For this review, take the finished solid that the model builds, in its own axes (mm). Face numbers are marked on the shaded views. A direction names the side the tool comes from. Coordinates: 2 decimals unless noted, no trailing zeros. Order: outer loops, then holes, each group sorted by start corner. A loop starts at its lowest first (then second) coordinate and runs counter-clockwise, first axis right, second up.
from build123d import *

# Parameters (mm, degrees)
SKETCH1_W                       = 100
SKETCH1_H                       = 100
BOSS_EXTRUDE1_DEPTH             = 95
SKETCH2_W                       = 10
SKETCH2_H                       = 10
BOSS_EXTRUDE2_DEPTH             = 105
SKETCH3_R                       = 1.4
CUT_EXTRUDE1_DEPTH              = 10
SKETCH4_W                       = 11
SKETCH4_H                       = 11
BOSS_EXTRUDE3_DEPTH             = 105
SKETCH5_R                       = 1.4
CUT_EXTRUDE2_DEPTH              = 10
SKETCH6_R                       = 1.4
CUT_EXTRUDE3_DEPTH              = 10
CHAMFER1_SIZE                   = 1
SKETCH7_W                       = 19
SKETCH7_H                       = 43
SKETCH7_W_2                     = 16
SKETCH7_H_2                     = 40
BOSS_EXTRUDE4_DEPTH             = 3
SKETCH8_W                       = 16
SKETCH8_H                       = 40
CUT_EXTRUDE4_DEPTH              = 10
CHAMFER2_SIZE                   = 13
SKETCH9_W                       = 16
SKETCH9_H                       = 3.1
CUT_EXTRUDE5_DEPTH              = 10
FILLET1_R                       = 1
SKETCH10_R                      = 1.4
CUT_EXTRUDE6_DEPTH              = 10
SKETCH12_W                      = 30.5
SKETCH12_H                      = 2.2
CUT_EXTRUDE7_DEPTH              = 3
SKETCH13_W                      = 30.5
SKETCH13_H                      = 2.2
CUT_EXTRUDE8_DEPTH              = 3
SKETCH14_W                      = 2.2
SKETCH14_H                      = 30.5
CUT_EXTRUDE9_DEPTH              = 3
CUT_EXTRUDE10_DEPTH             = 45
CUT_EXTRUDE10_DEPTH_BACK        = 45
SKETCH15_W                      = 90
SKETCH15_H                      = 58
CUT_EXTRUDE11_REACH             = 125.296
CUT_EXTRUDE11_DIRECTION_2_REACH = 125.296
CHAMFER3_SIZE                   = 4
CUT_EXTRUDE12_DEPTH             = 152.673992497
BOSS_EXTRUDE7_DEPTH             = 10
BOSS_EXTRUDE7_DEPTH_BACK        = 30.5
SKETCH19_W                      = 94
SKETCH19_H                      = 94
SKETCH19_W_2                    = 85
SKETCH19_H_2                    = 85
SKETCH20_R                      = 1.4
CUT_EXTRUDE13_DEPTH             = 123.316188626
SKETCH21_R                      = 1.4
CUT_EXTRUDE14_DEPTH             = 123.316188626
SKETCH22_W                      = 2.2
SKETCH22_H                      = 30.5
BOSS_EXTRUDE8_DEPTH             = 3
SKETCH23_R                      = 1.4
CUT_EXTRUDE15_DEPTH             = 20


with BuildPart() as part:
    # Sketch1 → Boss-Extrude1 (new body)
    with BuildSketch(Plane(origin=(0, 0, 0), x_dir=(1, 0, 0), z_dir=(0, 1, 0))):
        Rectangle(SKETCH1_W, SKETCH1_H)
    extrude(amount=BOSS_EXTRUDE1_DEPTH)

    # Sketch2 → Boss-Extrude2 (add)
    with BuildSketch(Plane(origin=(0, 100, 0), x_dir=(1, 0, 0), z_dir=(0, 1, 0))):
        with Locations((-45, 45)):
            Rectangle(SKETCH2_W, SKETCH2_H)
        with Locations((45, 45)):
            Rectangle(SKETCH2_W, SKETCH2_H)
        with Locations((45, -45)):
            Rectangle(SKETCH2_W, SKETCH2_H)
        with Locations((-45, -45)):
            Rectangle(SKETCH2_W, SKETCH2_H)
    extrude(amount=-BOSS_EXTRUDE2_DEPTH)

    # Sketch3 → Cut-Extrude1 (cut)
    with BuildSketch(Plane(origin=(0, 95, 0), x_dir=(1, 0, 0), z_dir=(0, 1, 0))):
        with Locations(Location((-28, -45, 0), (0, 0, 270))):
            Circle(SKETCH3_R)
        with Locations(Location((28, -45, 0), (0, 0, 90))):
            Circle(SKETCH3_R)
        with Locations(Location((28, 45, 0), (0, 0, 270))):
            Circle(SKETCH3_R)
        with Locations(Location((-28, 45, 0), (0, 0, 90))):
            Circle(SKETCH3_R)
    cut_extrude1 = extrude(amount=-CUT_EXTRUDE1_DEPTH, mode=Mode.SUBTRACT)

    # Sketch4 → Boss-Extrude3 (add)
    with BuildSketch(Plane(origin=(0, 100, 0), x_dir=(1, 0, 0), z_dir=(0, 1, 0))):
        with Locations((-45.5, 45.5)):
            Rectangle(SKETCH4_W, SKETCH4_H)
        with Locations((45.5, 45.5)):
            Rectangle(SKETCH4_W, SKETCH4_H)
        with Locations((45.5, -45.5)):
            Rectangle(SKETCH4_W, SKETCH4_H)
        with Locations((-45.5, -45.5)):
            Rectangle(SKETCH4_W, SKETCH4_H)
    extrude(amount=-BOSS_EXTRUDE3_DEPTH)

    # Sketch5 → Cut-Extrude2 (cut)
    with BuildSketch(Plane.XY.offset(50)):
        with Locations((-36, 91)):
            Circle(SKETCH5_R)
        with Locations(Location((36, 91, 0), (0, 0, 180))):
            Circle(SKETCH5_R)
        with Locations((36, 4)):
            Circle(SKETCH5_R)
        with Locations(Location((-36, 4, 0), (0, 0, 180))):
            Circle(SKETCH5_R)
    cut_extrude2 = extrude(amount=-CUT_EXTRUDE2_DEPTH, mode=Mode.SUBTRACT)

    # Mirror1: Cut-Extrude2 across plane
    add(cut_extrude2.mirror(Plane.XY), mode=Mode.SUBTRACT)

    # Sketch6 → Cut-Extrude3 (cut)
    with BuildSketch(Plane.ZY.offset(50)):
        with Locations((-36, 91)):
            Circle(SKETCH6_R)
        with Locations(Location((36, 91, 0), (0, 0, 180))):
            Circle(SKETCH6_R)
        with Locations((36, 4)):
            Circle(SKETCH6_R)
        with Locations(Location((-36, 4, 0), (0, 0, 180))):
            Circle(SKETCH6_R)
    cut_extrude3 = extrude(amount=-CUT_EXTRUDE3_DEPTH, mode=Mode.SUBTRACT)

    # Mirror2: Cut-Extrude3 across plane
    add(cut_extrude3.mirror(Plane(origin=(0, 0, 0), x_dir=(0, 0, 1), z_dir=(1, 0, 0))), mode=Mode.SUBTRACT)

    # Mirror3: Cut-Extrude1 across plane
    add(cut_extrude1.mirror(Plane.ZX.offset(47.5)), mode=Mode.SUBTRACT)

    # Chamfer1
    chamfer1_edges = [part.edges().sort_by_distance(p)[0] for p in [
        (-45.5, -5, 51),
        (-51, -5, 45.5),
        (-51, 100, 45.5),
        (-45.5, 100, 51),
        (51, -5, 45.5),
        (45.5, -5, 51),
        (45.5, 100, 51),
        (51, 100, 45.5),
        (45.5, -5, -51),
        (51, -5, -45.5),
        (51, 100, -45.5),
        (45.5, 100, -51),
        (-51, -5, -45.5),
        (-45.5, -5, -51),
        (-45.5, 100, -51),
        (-51, 100, -45.5),
        (-45.5, -5, 40),
        (-40, -5, 45.5),
        (-40, 100, 45.5),
        (-45.5, 100, 40),
        (40, -5, 45.5),
        (45.5, -5, 40),
        (45.5, 100, 40),
        (40, 100, 45.5),
        (45.5, -5, -40),
        (40, -5, -45.5),
        (45, 95, -40),
        (40, 100, -45.5),
        (45.5, 100, -40),
        (-40, -5, -45.5),
        (-45.5, -5, -40),
        (-45.5, 100, -40),
        (-40, 100, -45.5),
    ]]
    chamfer(chamfer1_edges, length=CHAMFER1_SIZE)

    # Sketch7 → Boss-Extrude4 (add)
    with BuildSketch(Plane(origin=(0, 95, 0), x_dir=(1, 0, 0), z_dir=(0, 1, 0))):
        with Locations((0, -17)):
            Rectangle(SKETCH7_W, SKETCH7_H)
        with Locations((0, -17)):
            Rectangle(SKETCH7_W_2, SKETCH7_H_2, mode=Mode.SUBTRACT)
    extrude(amount=BOSS_EXTRUDE4_DEPTH)

    # Sketch8 → Cut-Extrude4 (cut)
    with BuildSketch(Plane(origin=(0, 95, 0), x_dir=(1, 0, 0), z_dir=(0, 1, 0))):
        with Locations((0, -17)):
            Rectangle(SKETCH8_W, SKETCH8_H)
    extrude(amount=-CUT_EXTRUDE4_DEPTH, mode=Mode.SUBTRACT)

    # Chamfer2
    chamfer2_edges = [part.edges().sort_by_distance(p)[0] for p in [
        (0, 85, 37),
    ]]
    chamfer(chamfer2_edges, length=CHAMFER2_SIZE - 0.0001)  # a hair under: the kernel refuses the full size

    # Sketch9 → Cut-Extrude5 (cut)
    with BuildSketch(Plane(origin=(0, 85, 0), x_dir=(1, 0, 0), z_dir=(0, 1, 0))):
        with Locations((0, 1.45)):
            Rectangle(SKETCH9_W, SKETCH9_H)
    extrude(amount=-CUT_EXTRUDE5_DEPTH, mode=Mode.SUBTRACT)

    # Fillet1
    fillet1_edges = [part.edges().sort_by_distance(p)[0] for p in [
        (0, 85, 0.1),
    ]]
    fillet(fillet1_edges, radius=FILLET1_R)

    # Sketch10 → Cut-Extrude6 (cut)
    with BuildSketch(Plane.XY.offset(-3)):
        with Locations((0, 92)):
            Circle(SKETCH10_R)
    extrude(amount=-CUT_EXTRUDE6_DEPTH, mode=Mode.SUBTRACT)

    # Sketch12 → Cut-Extrude7 (cut)
    with BuildSketch(Plane.ZY.offset(50)):
        with Locations((0, 74.4)):
            Rectangle(SKETCH12_W, SKETCH12_H)
        with Locations((0, 20.6)):
            Rectangle(SKETCH12_W, SKETCH12_H)
    cut_extrude7 = extrude(amount=-CUT_EXTRUDE7_DEPTH, mode=Mode.SUBTRACT)

    # Mirror4: Cut-Extrude7 across plane
    add(cut_extrude7.mirror(Plane(origin=(0, 0, 0), x_dir=(0, 0, 1), z_dir=(1, 0, 0))), mode=Mode.SUBTRACT)

    # Sketch13 → Cut-Extrude8 (cut)
    with BuildSketch(Plane.XY.offset(50)):
        with Locations((0, 74.4)):
            Rectangle(SKETCH13_W, SKETCH13_H)
        with Locations((0, 20.6)):
            Rectangle(SKETCH13_W, SKETCH13_H)
    cut_extrude8 = extrude(amount=-CUT_EXTRUDE8_DEPTH, mode=Mode.SUBTRACT)

    # Mirror5: Cut-Extrude8 across plane
    add(cut_extrude8.mirror(Plane.XY), mode=Mode.SUBTRACT)

    # Sketch14 → Cut-Extrude9 (cut)
    with BuildSketch(Plane(origin=(0, 95, 0), x_dir=(1, 0, 0), z_dir=(0, 1, 0))):
        with Locations((26.9, 0)):
            Rectangle(SKETCH14_W, SKETCH14_H)
        with Locations((-26.9, 0)):
            Rectangle(SKETCH14_W, SKETCH14_H)
    cut_extrude9 = extrude(amount=-CUT_EXTRUDE9_DEPTH, mode=Mode.SUBTRACT)

    # Mirror6: Cut-Extrude9 across plane
    add(cut_extrude9.mirror(Plane.ZX.offset(47.5)), mode=Mode.SUBTRACT)

    # Sketch15 → Cut-Extrude10 (cut, two sides: drawn at the far end of the back side and taken through both)
    with BuildSketch(Plane(origin=(0, 0, 0), x_dir=(0, 0, -1), z_dir=(1, 0, 0)).offset(-CUT_EXTRUDE10_DEPTH_BACK)):
        with Locations((0, 41)):
            Rectangle(SKETCH15_W, SKETCH15_H)
    extrude(amount=CUT_EXTRUDE10_DEPTH + CUT_EXTRUDE10_DEPTH_BACK, mode=Mode.SUBTRACT)

    # Cut-Extrude11: up to this face of the body (flat: up to its plane)
    cut_extrude11_end = Plane(part.part.faces().sort_by_distance((0, 41, 45))[0])
    # Sketch16 → Cut-Extrude11 (cut, up to the picked face)
    with BuildSketch(Plane.XY, mode=Mode.PRIVATE) as cut_extrude11_sk1:
        Polygon((45, 57.006357685), (-45, 57.006357685), (-45, 83), (-13, 83), (-13, 67.006357685), (13, 67.006357685), (13, 83), (45, 83), align=None)
    cut_extrude11_tool1 = split(extrude(cut_extrude11_sk1.sketch, amount=CUT_EXTRUDE11_REACH, mode=Mode.PRIVATE), bisect_by=cut_extrude11_end, keep=Keep.BOTH, mode=Mode.PRIVATE)
    add(cut_extrude11_tool1.solids().sort_by(Axis((0, 57.943143, 0), (0, 0, 1)))[0], mode=Mode.SUBTRACT)

    # Cut-Extrude11 direction 2: up to this face of the body (flat: up to its plane)
    cut_extrude11_direction_2_end = Plane(part.part.faces().sort_by_distance((0, 41, -45))[0])
    # Sketch16 → Cut-Extrude11 direction 2 (cut, up to the picked face)
    with BuildSketch(Plane.XY, mode=Mode.PRIVATE) as cut_extrude11_direction_2_sk1:
        Polygon((45, 57.006357685), (-45, 57.006357685), (-45, 83), (-13, 83), (-13, 67.006357685), (13, 67.006357685), (13, 83), (45, 83), align=None)
    cut_extrude11_direction_2_tool1 = split(extrude(cut_extrude11_direction_2_sk1.sketch, amount=-CUT_EXTRUDE11_DIRECTION_2_REACH, mode=Mode.PRIVATE), bisect_by=cut_extrude11_direction_2_end, keep=Keep.BOTH, mode=Mode.PRIVATE)
    add(cut_extrude11_direction_2_tool1.solids().sort_by(Axis((0, 57.943143, 0), (0, 0, -1)))[0], mode=Mode.SUBTRACT)

    # Chamfer3
    chamfer3_edges = [part.edges().sort_by_distance(p)[0] for p in [
        (13, 70, 0),
        (-13, 70, 0),
    ]]
    chamfer(chamfer3_edges, length=CHAMFER3_SIZE)

    # Sketch17 → Cut-Extrude12 (cut, through all)
    with BuildSketch(Plane(origin=(0, 0, -51), x_dir=(-1, 0, 0), z_dir=(0, 0, -1))):
        Polygon((-51, 47.5), (-51, 104.912758391), (51, 104.912758391), (51, 47.5), (51, 42.5), (-51, 42.5), align=None)
    extrude(amount=-CUT_EXTRUDE12_DEPTH, mode=Mode.SUBTRACT)

    # Sketch19 → Boss-Extrude7 (add, two sides: drawn at the far end of the back side and taken through both)
    with BuildSketch(Plane(origin=(0, 42.5, 0), x_dir=(1, 0, 0), z_dir=(0, 1, 0)).offset(-BOSS_EXTRUDE7_DEPTH_BACK)):
        Rectangle(SKETCH19_W, SKETCH19_H)
        Rectangle(SKETCH19_W_2, SKETCH19_H_2, mode=Mode.SUBTRACT)
    extrude(amount=BOSS_EXTRUDE7_DEPTH + BOSS_EXTRUDE7_DEPTH_BACK)

    # Sketch20 → Cut-Extrude13 (cut, through all)
    with BuildSketch(Plane.XY.offset(47)):
        with Locations((0, 47.5)):
            Circle(SKETCH20_R)
    extrude(amount=-CUT_EXTRUDE13_DEPTH, mode=Mode.SUBTRACT)

    # Sketch21 → Cut-Extrude14 (cut, through all)
    with BuildSketch(Plane(origin=(47, 0, 0), x_dir=(0, 0, -1), z_dir=(1, 0, 0))):
        with Locations((0, 47.5)):
            Circle(SKETCH21_R)
    extrude(amount=-CUT_EXTRUDE14_DEPTH, mode=Mode.SUBTRACT)

    # Sketch22 → Boss-Extrude8 (add)
    with BuildSketch(Plane.XZ):
        with Locations((26.9, 0)):
            Rectangle(SKETCH22_W, SKETCH22_H)
        with Locations((-26.9, 0)):
            Rectangle(SKETCH22_W, SKETCH22_H)
    extrude(amount=-BOSS_EXTRUDE8_DEPTH)

    # Sketch23 → Cut-Extrude15 (cut)
    with BuildSketch(Plane.XZ):
        with Locations(Location((-40, 0, 0), (0, 0, 270))):
            Circle(SKETCH23_R)
        with Locations(Location((0, 40, 0), (0, 0, 270))):
            Circle(SKETCH23_R)
        with Locations(Location((40, 0, 0), (0, 0, 270))):
            Circle(SKETCH23_R)
        with Locations(Location((0, -40, 0), (0, 0, 270))):
            Circle(SKETCH23_R)
    extrude(amount=-CUT_EXTRUDE15_DEPTH, mode=Mode.SUBTRACT)


solid = part.part
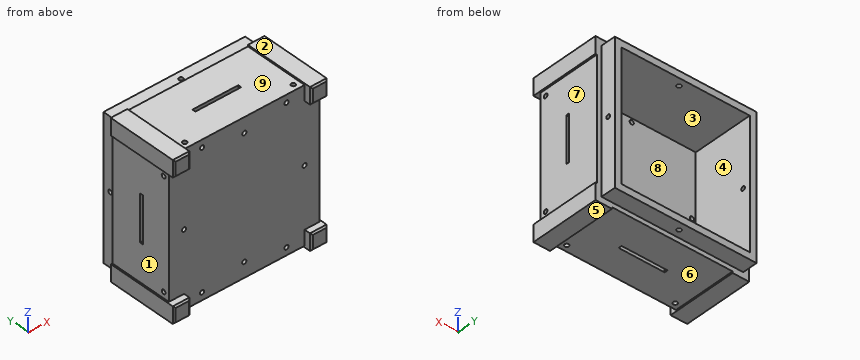
1. Clearance check with flat-ended pins moving along their axes: pin 1 Ø11 at (x, y) = (-18.5, 46) entering from +Z; pin 2 Ø0.8 at (y, z) = (4.5, -35.5) entering from -X; pin 3 Ø5 at (y, z) = (18, -14) entering from +X; pin 4 Ø2.5 at (x, y) = (0, 47.5) entering from -Z. State where each tip first meets the part, or that it passes through.
Answer below:
pin 1: stops at z = 50
pin 2: stops at x = -40
pin 3: stops at x = 50
pin 4: passes through
2. Take a section at D-D, the plane y = 33.5. Give the boundary of the cut face in (x, z).
Answer below:
outline: (-51, -51) - (-40, -51) - (-40, -50) - (40, -50) - (40, -51) - (51, -51) - (51, -40) - (50, -40) - (50, 40) - (51, 40) - (51, 51) - (40, 51) - (40, 50) - (-40, 50) - (-40, 51) - (-51, 51) - (-51, 40) - (-50, 40) - (-50, -40) - (-51, -40) - close; hole (-42.5, -42.5) - (42.5, -42.5) - (42.5, 42.5) - (-42.5, 42.5) - close
3. Take a section at C-C, the plane x = -36. Give the boundary of the cut face in (y, z), plus the area to 3 significant figures.
Answer below:
outline: (0, -50) - (2.6, -50) - (2.6, -40) - (5.4, -40) - (5.4, -50) - (42.5, -50) - (42.5, -47) - (52.5, -47) - (52.5, -42.5) - (12, -42.5) - (12, 42.5) - (52.5, 42.5) - (52.5, 47) - (42.5, 47) - (42.5, 50) - (5.4, 50) - (5.4, 40) - (2.6, 40) - (2.6, 50) - (0, 50) - close
area: 1,690 mm2
4. Take a section at A-A, the plane y = 8. Give the number of separate pieces and of enclosed holes in the cut face, plus the area to 3 significant figures.
Answer below:
separate pieces: 1
enclosed holes: 8
area: 10,000 mm2
5. To check wall thickness, follow L1, parallel to X at y = 7, z = -45; L2, parallel to Y at x = 0, z = 44; L3, parallel to Z at x = -13, y = 26.5. State the ranges of each line that lie inside material, in increasing order.
Answer below:
L1: x = -51 to -29.4, -26.6 to 26.6, 29.4 to 51
L2: y = 0 to 46.1, 48.9 to 52.5
L3: z = -50 to -42.5, 42.5 to 50
6. Take a section at B-B, the plane z = -36. Give the boundary of the cut face in (x, y), plus the area to 3 significant figures.
Answer below:
outline: (-50, 0) - (50, 0) - (50, 2.6) - (40, 2.6) - (40, 5.4) - (50, 5.4) - (50, 42.5) - (47, 42.5) - (47, 52.5) - (42.5, 52.5) - (42.5, 12) - (-42.5, 12) - (-42.5, 52.5) - (-47, 52.5) - (-47, 42.5) - (-50, 42.5) - (-50, 5.4) - (-40, 5.4) - (-40, 2.6) - (-50, 2.6) - close
area: 1,690 mm2
7. The part is to be moulded in two halves that separate along X. For the marked faces 1, 2, 3 and 4, say which applies: +X half, -X half, draft (parallel to the pull), parting line (faces both ways), or undercut.
Answer below:
face 1: -X half
face 2: draft
face 3: undercut
face 4: undercut
8. Machinability: for the marked faces 5, 6, 7, 8 and 9, which of the approach directions +Z, -Z, +X, -X, +Y, -Y give a long, thin tool a straight path to every point of the face, cutting with its end or side? Answer none if there is none.
Answer below:
face 5: -Z, +X, -X, +Y, -Y
face 6: -Z, +Y, -Y
face 7: +X, +Y, -Y
face 8: +Y
face 9: +Z, +Y, -Y
